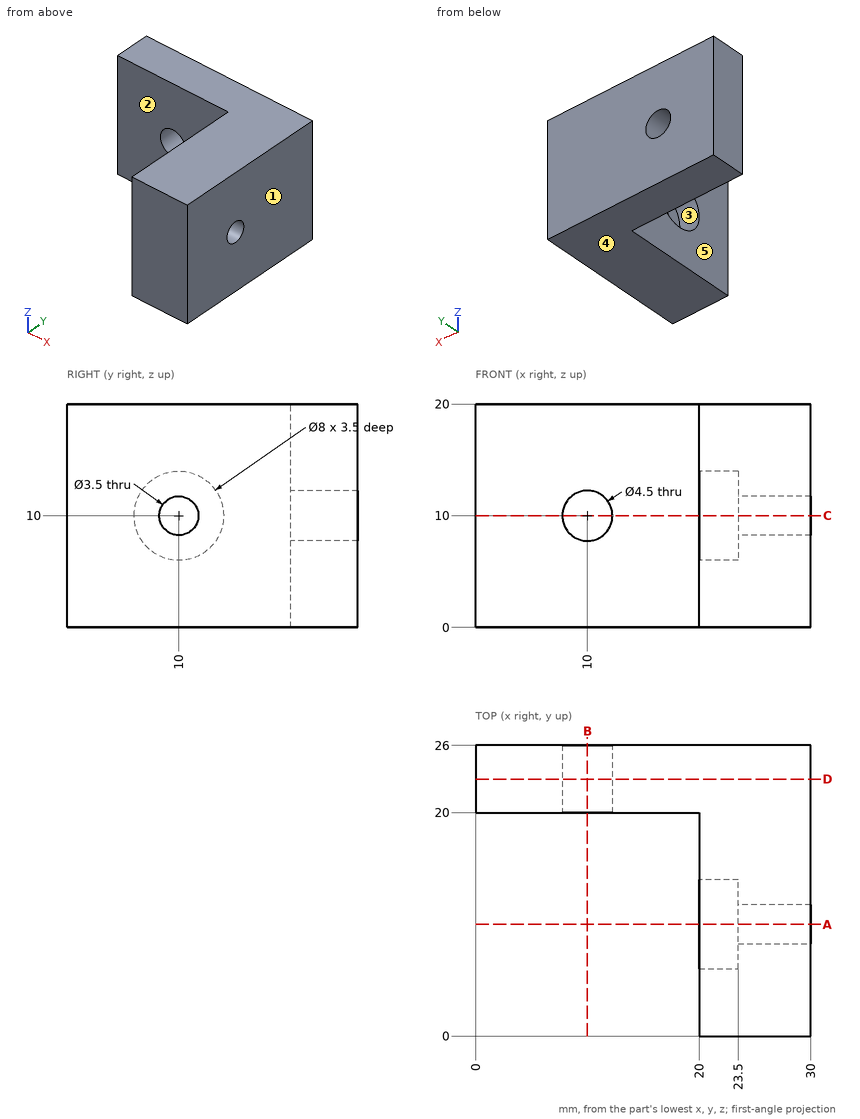
The figure shows three views and two pictorial views of one solid part (mm, origin at its lowest corner). Answer the questions. A direction names the side the tool comes from. Round coordinates to 2 decimals unless told otherwise and drop trailing zeros. Order: outer loops, then holes, each group sorted by start corner. A loop starts at its lowest first (then second) coordinate and runs counter-clockwise, first axis right, second up.
Q1. The mould has two halves that part along Z. Classify the marked faces 3, 4 and 5: pulls with the +Z half, pulls with the -Z half, needs draft (parallel to the pull), parting line crosses it, or undercut.
Solution:
face 3: undercut
face 4: pulls with the -Z half
face 5: needs draft
Q2. Find the intervals of material crossed by line 1 along Z through (x, y) = (10, 21.55); line 2 along Z through (x, y) = (27, 10); line 3 along X through (y, z) = (13.5, 19), in increasing order.
Solution:
line 1: z = 0 to 7.75, 12.25 to 20
line 2: z = 0 to 8.25, 11.75 to 20
line 3: x = 20 to 30
Q3. A cutting plane is placed at A-A, the plane y = 10. Determine the outline of the cut face in (x, z).
Solution:
outline: (20, 0) - (30, 0) - (30, 8.25) - (23.5, 8.25) - (23.5, 6) - (20, 6) - close; (20, 14) - (23.5, 14) - (23.5, 11.75) - (30, 11.75) - (30, 20) - (20, 20) - close
Q4. A tool of negligible diameter and unlimited length cuts with its end or side. For the marked faces 1 and 2, from which of +Z, -Z, +X, -X, +Y, -Y can it reach the whole face along a straight path? Write none if from no direction.
Solution:
face 1: +Z, -Z, +X, +Y, -Y
face 2: +Z, -Z, -X, -Y
Q5. Given pin 1 Ø3 at (y, z) = (14.5, 10.5) entering from -X; pin 2 Ø6 at (x, z) = (5.5, 9.5) entering from -Y, each flat-ended and moving along its own axis, determine where each tip first touches the part or whether it passes through.
Solution:
pin 1: stops at x = 20
pin 2: stops at y = 20
Q6. A cutting plane is placed at B-B, the plane x = 10. Determine the outline of the cut face in (y, z).
Solution:
outline: (20, 0) - (26, 0) - (26, 7.75) - (20, 7.75) - close; (20, 12.25) - (26, 12.25) - (26, 20) - (20, 20) - close
Q7. A cutting plane is placed at C-C, the plane z = 10. Determine the outline of the cut face in (x, y).
Solution:
outline: (0, 20) - (7.75, 20) - (7.75, 26) - (0, 26) - close; (12.25, 20) - (20, 20) - (20, 14) - (23.5, 14) - (23.5, 11.75) - (30, 11.75) - (30, 26) - (12.25, 26) - close; (20, 0) - (30, 0) - (30, 8.25) - (23.5, 8.25) - (23.5, 6) - (20, 6) - close
Q8. A cutting plane is placed at D-D, the plane y = 23. Determine the outline of the cut face in (x, z).
Solution:
outline: (0, 0) - (30, 0) - (30, 20) - (0, 20) - close; hole circle Ø4.5 at (10, 10)
